Here's how the part is built. I have some questions about the finished solid (model axes, mm). A direction names the side the tool comes from. Round coordinates to 2 decimals unless told otherwise and drop trailing zeros. Write each loop counter-clockwise with the first axis right and the second up, starting at its lowest first coordinate (ties: lowest second). Pieces come first, ordered by that corner, then holes. Notation, with made-up numbers: M 39.5,48 L 78.5,48 A27 cw 78.5,71 Z; hole C -21.75,-2 d8. An arc over 180 degrees is marked long. Write item = value, one per line. Start each with the question number.
(1) Will these pins go through, and if not, where does the flat tip stop? pin 1 Ø10 at (x, y) = (-3, 44) entering from -Z; pin 2 Ø1 at (y, z) = (70.5, 1.5) entering from +X; pin 3 Ø1 at (x, z) = (31, 1.5) entering from +Y.
(2) If we mould it in two halves opening along Y, with no side actions, what happens to faces 3 (the cylindrical face through (-1.86, 64.966, 1.565)), 4 (the flat face through (33, -12.7, 2)), 5 (the flat face through (33, 63.5, 2))? For each: released by +Y, released by -Y, zero draft, split by the parting line, or undercut.
(3) I want a section at A-A (y = 25.4). List the corners of the cut face in (x, z) for me (3 decimals), and give its area (3 significant figures).
(4) I want a section at C-C (y = 12.7). List the corners of the cut face in (x, z) for me (3 decimals), and give its area (3 significant figures).
(5) I need wall thicknesses on line 1 along Y through (x, z) = (0, 1.3); line 2 along Y through (x, z) = (38.1, 0.9); line 3 along Y through (x, z) = (18, 0.9). Which ranges of each line are inside material? Lowest first, please.
(6) I want a section at B-B (x = 0). List the corners of the cut face in (y, z) for me (1 decimal), and give its area (3 significant figures).
(7) On a 3-axis mill with a long thin cutter (end or side, diameter ignored), from which of +Z, -Z, +X, -X, +Y, -Y can I reach the whole of each face in a straight line? I mean faces 1 (the flat face through (25.4, 70, 2)), 2 (the cylindrical face through (46.98, -9.08, 1.57)). Say none if no direction works.
(8) I want a section at D-D (z = 1.4). Give the number of separate pieces and of enclosed holes in the cut face, and give its area (3 significant figures).
```python
from build123d import *

# Parameters (mm, degrees)
SKETCH1_R           = 1.9939
SKETCH1_R_2         = 14.2875
BOSS_EXTRUDE1_DEPTH = 3.175
FILLET1_R           = 2.54


with BuildPart() as part:
    # Sketch1 → Boss-Extrude1 (new body)
    with BuildSketch(Plane.XY):
        with BuildLine():
            Line((25.4, 76.2), (-31.75, 76.2))
            Line((-31.75, 76.2), (-31.75, -25.4))
            Line((-31.75, -25.4), (25.4, -25.4))
            Line((25.4, -25.4), (25.4, -12.7))
            Line((25.4, -12.7), (38.1, -12.7))
            ThreePointArc((38.1, -12.7), (47.080256121, -8.980256121), (50.8, 0))
            Line((50.8, 0), (50.8, 50.8))
            ThreePointArc((50.8, 50.8), (47.080256121, 59.780256121), (38.1, 63.5))
            Line((38.1, 63.5), (25.4, 63.5))
            Line((25.4, 63.5), (25.4, 76.2))
        make_face()
        with Locations((-18.034, -18.034)):
            Circle(SKETCH1_R, mode=Mode.SUBTRACT)
        with Locations((-18.034, 18.034)):
            Circle(SKETCH1_R, mode=Mode.SUBTRACT)
        Circle(SKETCH1_R_2, mode=Mode.SUBTRACT)
        with Locations((18.034, -18.034)):
            Circle(SKETCH1_R, mode=Mode.SUBTRACT)
        with Locations((18.034, 18.034)):
            Circle(SKETCH1_R, mode=Mode.SUBTRACT)
        with Locations((38.1, 0)):
            Circle(SKETCH1_R, mode=Mode.SUBTRACT)
        with Locations((38.1, 12.7)):
            Circle(SKETCH1_R, mode=Mode.SUBTRACT)
        with Locations((0, 50.8)):
            Circle(SKETCH1_R_2, mode=Mode.SUBTRACT)
        with Locations((38.1, 25.4)):
            Circle(SKETCH1_R, mode=Mode.SUBTRACT)
        with Locations((38.1, 38.1)):
            Circle(SKETCH1_R, mode=Mode.SUBTRACT)
        with Locations((38.1, 50.8)):
            Circle(SKETCH1_R, mode=Mode.SUBTRACT)
    extrude(amount=BOSS_EXTRUDE1_DEPTH)

    # Fillet1
    fillet1_edges = [part.edges().sort_by_distance(p)[0] for p in [
        (25.4, -12.7, 1.5875),
        (25.4, -25.4, 1.5875),
        (-31.75, -25.4, 1.5875),
        (-31.75, 76.2, 1.5875),
        (25.4, 76.2, 1.5875),
        (25.4, 63.5, 1.5875),
    ]]
    fillet(fillet1_edges, radius=FILLET1_R)


solid = part.part
```
Returned:
q1.pin_1 = through
q1.pin_2 = 25.4
q1.pin_3 = 63.5
q2.face_3 = undercut
q2.face_4 = released by -Y
q2.face_5 = released by +Y
q3.outline = M -31.75,0 L 36.106,0 L 36.106,3.175 L -31.75,3.175 Z; M 40.094,0 L 50.8,0 L 50.8,3.175 L 40.094,3.175 Z
q3.area = 249 mm²
q4.outline = M -31.75,0 L -6.545,0 L -6.545,3.175 L -31.75,3.175 Z; M 6.545,0 L 36.106,0 L 36.106,3.175 L 6.545,3.175 Z; M 40.094,0 L 50.8,0 L 50.8,3.175 L 40.094,3.175 Z
q4.area = 208 mm²
q5.line_1 = -25.4 to -14.29, 14.29 to 36.51, 65.09 to 76.2
q5.line_2 = -12.7 to -1.99, 1.99 to 10.71, 14.69 to 23.41, 27.39 to 36.11, 40.09 to 48.81, 52.79 to 63.5
q5.line_3 = -25.4 to -20.03, -16.04 to 16.04, 20.03 to 76.2
q6.outline = M -25.4,0 L -14.3,0 L -14.3,3.2 L -25.4,3.2 Z; M 14.3,0 L 36.5,0 L 36.5,3.2 L 14.3,3.2 Z; M 65.1,0 L 76.2,0 L 76.2,3.2 L 65.1,3.2 Z
q6.area = 141 mm²
q7.face_1 = +Z, -Z, +X, +Y
q7.face_2 = +Z, -Z, +X, -Y
q8.separate_pieces = 1
q8.enclosed_holes = 11
q8.area = 6,270 mm²
